Can you work these out from the drawing? Everything is in mm from the part's minimum corner. Give positions to 0.01 mm unless a question says otherwise; leave off trailing zeros. Order: outer loops, then holes, each group sorted by start corner. A loop starts at its lowest first (then second) coordinate and runs counter-clockwise, first axis right, second up. Notation, with made-up numbers: (-8.75, -39.75) - (-2.75, -39.75) arc R28 cw to (-2.75, -12.75) - close; hole circle Ø10 at (-0.75, 28). An arc over 180 degrees is marked (long way). Answer as a JSON object with one key per item and string values.
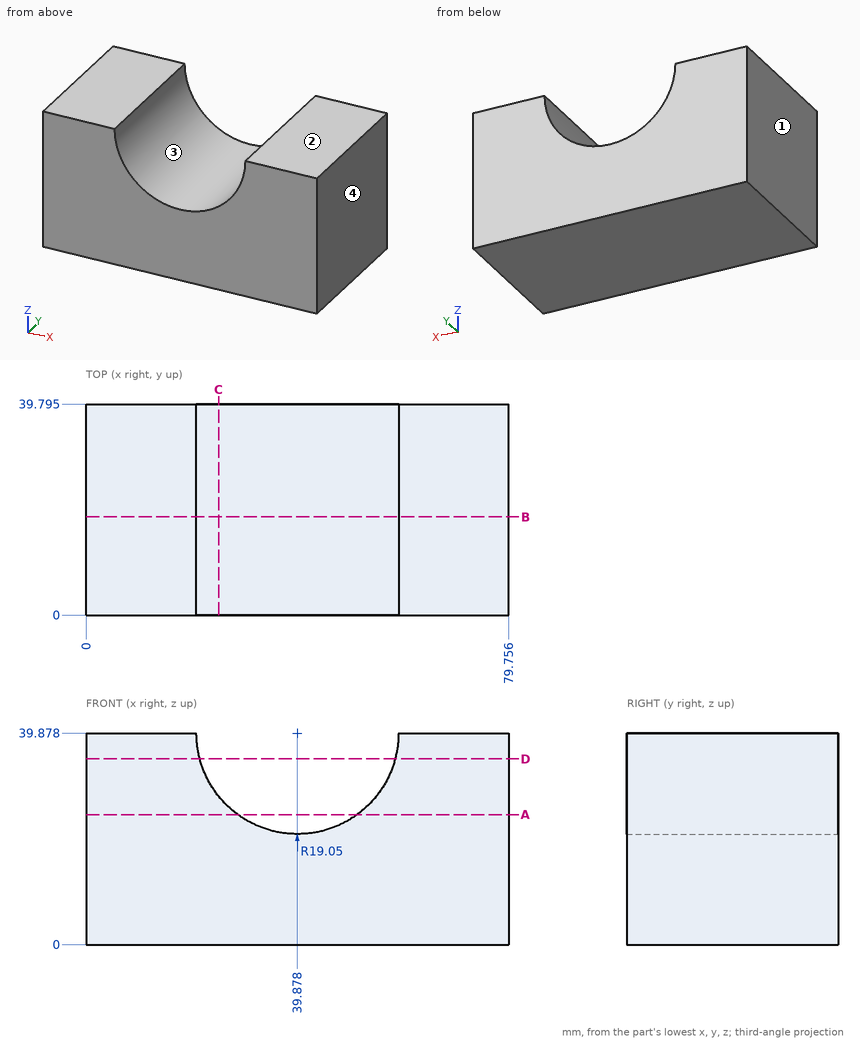
Q1. We'd pull the mould along X, two halves only. Please class the marked faces 1, 2, 3 and 4: released by +X, released by -X, zero draft, split by the parting line, or undercut.
Recorded:
{"face 1": "released by -X", "face 2": "zero draft", "face 3": "undercut", "face 4": "released by +X"}
Q2. If we section it at A-A, the plane z = 24.5: Please give me the cut outline in (x, y) (1 decimal).
Recorded:
{"outline": "(0, 0) - (28.6, 0) - (28.6, 39.8) - (0, 39.8) - close; (51.1, 0) - (79.8, 0) - (79.8, 39.8) - (51.1, 39.8) - close"}
Q3. If we section it at B-B, the plane y = 18.5: Please give me the cut outline in (x, z).
Recorded:
{"outline": "(0, 0) - (79.76, 0) - (79.76, 39.88) - (58.93, 39.88) arc R19.05 cw to (20.83, 39.88) - (0, 39.88) - close"}
Q4. I need wall thicknesses on L1, parallel to X at y = 27, z = 23 (1 decimal); L2, parallel to X at y = 14, z = 34; L3, parallel to Z at x = 23.5, y = 6. Which ranges of each line are inside material? Lowest first, please.
Recorded:
{"L1": "x = 0 to 31, 48.7 to 79.8", "L2": "x = 0 to 21.76, 58 to 79.76", "L3": "z = 0 to 30.15"}
Q5. If we section it at D-D, the plane z = 35: Please give me the cut outline in (x, y) (3 decimals), then the cut area to 3 significant figures.
Recorded:
{"outline": "(0, 0) - (21.463, 0) - (21.463, 39.795) - (0, 39.795) - close; (58.293, 0) - (79.756, 0) - (79.756, 39.795) - (58.293, 39.795) - close", "area": "1,710 mm^2"}
Q6. I'm going to push a flat-ended pin straight in: pin 1 Ø3 at (x, y) = (44.5, 20) entering from +Z. Where does the tip first touch, or does it pass through?
Recorded:
{"pin 1": "stops at z = 21.84"}
Q7. If we section it at C-C, the plane x = 25: Please give me the cut outline in (y, z) (1 decimal).
Recorded:
{"outline": "(0, 0) - (39.8, 0) - (39.8, 28) - (0, 28) - close"}
